Source: CAD feature listing. Evaluate the final solid. Frame: model axes, mm. A direction names the side the tool comes from. Give positions to 0.01 mm unless a question says otherwise; leave off trailing zeros. Order: outer loops, then holes, each group sorted by start corner. A loop starts at its lowest first (then second) coordinate and runs counter-clockwise, first axis right, second up. Notation, with made-up numbers: (61, 4.5) -> (107, 4.5) arc R10 cw to (107, 22.5) -> close; hole circle Ø9 at (42, 1). An arc over 180 degrees is marked (long way). Answer in a Markdown table with one row per item.
```python
from build123d import *

# Parameters (mm, degrees)
F1_DEPTH     = 76.2
F2_R         = 50.0828504331
F2_R_2       = 13.7976444657
F3_DEPTH     = 50.8
F4_T         = -2.54
F5_T3_DEPTH  = 203.2
F5_T5_DEPTH  = 203.2
F5_T8_ANGLE  = 208.0724869359
F5_T10_ANGLE = 151.9275130641


# Not quite as in the source:
# - a fillet or chamfer that OpenCascade refuses, or shapes differently, is made with other operations: its cross-section is extruded or revolved along the edge and cut away or added


with BuildPart() as f1:
    # F0 (on Right) → F1 (new body)
    with BuildSketch(Plane.YZ):
        with BuildLine():
            ThreePointArc((18.4812146278, -73.9248585111), (60.0612543768, -46.8944103565), (76.2, 0))
            ThreePointArc((76.2, 0), (60.0612543768, 46.8944103565), (18.4812146278, 73.9248585111))
            ThreePointArc((18.4812146278, 73.9248585111), (-76.2, 0), (18.4812146278, -73.9248585111))
        make_face()
        with BuildLine():
            ThreePointArc((18.4812146278, 73.9248585111), (60.0612543768, 46.8944103565), (76.2, 0))
            ThreePointArc((76.2, 0), (60.0612543768, -46.8944103565), (18.4812146278, -73.9248585111))
            Line((18.4812146278, -73.9248585111), (215.6141706573, -24.6416195037))
            ThreePointArc((215.6141706573, -24.6416195037), (184.0537657814, 0), (215.6141706573, 24.6416195037))
            Line((215.6141706573, 24.6416195037), (18.4812146278, 73.9248585111))
        make_face()
        with BuildLine():
            ThreePointArc((234.8537657814, 0), (229.474183907, 15.6314701188), (215.6141706573, 24.6416195037))
            ThreePointArc((215.6141706573, 24.6416195037), (184.0537657814, 0), (215.6141706573, -24.6416195037))
            ThreePointArc((215.6141706573, -24.6416195037), (229.474183907, -15.6314701188), (234.8537657814, 0))
        make_face()
    extrude(amount=F1_DEPTH)

    # F2 (on face) → F3 (cut)
    with BuildSketch(Plane.YZ.offset(76.2)):
        Circle(F2_R)
        with Locations((209.4537657814, 0)):
            Circle(F2_R_2)
    extrude(amount=-F3_DEPTH, mode=Mode.SUBTRACT)

    # F4
    f4_openings = [f1.faces().sort_by_distance(p)[0] for p in [
        (0, 57.51924, 0),
    ]]
    offset(amount=F4_T, openings=f4_openings, kind=Kind.INTERSECTION)

    # F5: fillet of radius 6.35 on 7 edges, made by hand

    # F5_s1 → F5_t2 (revolve)
    with BuildSketch(Plane.XY):
        with BuildLine():
            ThreePointArc((31.75, 50.0828504331), (27.2598719395, 48.2229784936), (25.4, 43.7328504331))
            Line((25.4, 43.7328504331), (25.4, 50.0828504331))
            Line((25.4, 50.0828504331), (31.75, 50.0828504331))
        make_face()
    revolve(axis=Axis((25.4, 0, 0), (1, 0, 0)))

    # F5_s4 → F5_t3 (cut)
    with BuildSketch(Plane(origin=(0, 197.1329560295, -49.2832390074), x_dir=(1, 0, 0), z_dir=(0, -0.9701425001, 0.242535625))):
        with BuildLine():
            ThreePointArc((69.85, 76.2), (74.3401280605, 74.3401280605), (76.2, 69.85))
            Line((76.2, 69.85), (76.2, 76.2))
            Line((76.2, 76.2), (69.85, 76.2))
        make_face()
    extrude(amount=F5_T3_DEPTH, mode=Mode.SUBTRACT)

    # F5_s6 → F5_t5 (cut)
    with BuildSketch(Plane(origin=(0, 0, 0), x_dir=(1, 0, 0), z_dir=(0, 0.9701425001, 0.242535625))):
        with BuildLine():
            ThreePointArc((69.85, 76.2), (74.3401280605, 74.3401280605), (76.2, 69.85))
            Line((76.2, 69.85), (76.2, 76.2))
            Line((76.2, 76.2), (69.85, 76.2))
        make_face()
    extrude(amount=F5_T5_DEPTH, mode=Mode.SUBTRACT)

    # F5_s7 → F5_t8 (revolve, cut)
    with BuildSketch(Plane(origin=(0, 0, 0), x_dir=(1, 0, 0), z_dir=(0, 0.9701425001, -0.242535625))):
        with BuildLine():
            ThreePointArc((69.85, -76.2), (74.3401280605, -74.3401280605), (76.2, -69.85))
            Line((76.2, -69.85), (76.2, -76.2))
            Line((76.2, -76.2), (69.85, -76.2))
        make_face()
    revolve(axis=Axis((76.2, 0, 0), (1, 0, 0)), revolution_arc=F5_T8_ANGLE, mode=Mode.SUBTRACT)

    # F5_s9 → F5_t10 (revolve, cut)
    with BuildSketch(Plane(origin=(0, 197.1329560295, 49.2832390074), x_dir=(1, 0, 0), z_dir=(0, -0.9701425001, -0.242535625))):
        with BuildLine():
            ThreePointArc((76.2, -69.85), (74.3401280605, -74.3401280605), (69.85, -76.2))
            Line((69.85, -76.2), (76.2, -76.2))
            Line((76.2, -76.2), (76.2, -69.85))
        make_face()
    revolve(axis=Axis((76.2, 209.4537657814, 0), (1, 0, 0)), revolution_arc=F5_T10_ANGLE, mode=Mode.SUBTRACT)

    # F5_s11 → F5_t12 (revolve, cut)
    with BuildSketch(Plane.XY):
        with BuildLine():
            ThreePointArc((76.2, 56.4328504331), (74.3401280605, 51.9427223726), (69.85, 50.0828504331))
            Line((69.85, 50.0828504331), (76.2, 50.0828504331))
            Line((76.2, 50.0828504331), (76.2, 56.4328504331))
        make_face()
    revolve(axis=Axis((76.2, 0, 0), (1, 0, 0)), mode=Mode.SUBTRACT)

    # F5_s13 → F5_t14 (revolve, cut)
    with BuildSketch(Plane.XY):
        with BuildLine():
            ThreePointArc((76.2, 229.6014102471), (74.3401280605, 225.1112821866), (69.85, 223.2514102471))
            Line((69.85, 223.2514102471), (76.2, 223.2514102471))
            Line((76.2, 223.2514102471), (76.2, 229.6014102471))
        make_face()
    revolve(axis=Axis((76.2, 209.4537657814, 0), (1, 0, 0)), mode=Mode.SUBTRACT)


solid = f1.part
```
(1) Pull-direction query (Y, two-part tool) for faces 1 (the flat face through (0, 79, 57)), 2 (the flat face through (36.314, 115.052, -47.164)), 3 (the flat face through (34.436, 115.668, -49.628)); classes: +Y half, -Y half, draft (parallel to the pull), parting line (faces both ways), or undercut.
A:
| item | result |
|---|---|
| face 1 | draft |
| face 2 | undercut |
| face 3 | +Y half |
(2) Access query for faces 4 (the flat face through (36.314, 117.812, 46.474)), 5 (the cylindrical face through (47.94, 195.67, 0.61)), 6 (the cylindrical face through (74.29, 115.23, -47.87)). Directions: +Z, -Z, +X, -X, +Y, -Y. A direction counts if a zero-diameter tool reaches every point of the face in a straight line with its end or side. Return the directions, or none.
A:
| item | result |
|---|---|
| face 4 | -X |
| face 5 | +X |
| face 6 | -Z, +X, +Y |
(3) Section query C-C (y = 0). Return the cut outline in (x, z).
A:
| item | result |
|---|---|
| outline | (0, -76.2) -> (69.85, -76.2) arc R6.35 ccw to (76.2, -69.85) -> (76.2, -56.43) arc R6.35 ccw to (69.85, -50.08) -> (31.75, -50.08) arc R6.35 cw to (25.4, -43.73) -> (25.4, 43.73) arc R6.35 cw to (31.75, 50.08) -> (69.85, 50.08) arc R6.35 ccw to (76.2, 56.43) -> (76.2, 69.85) arc R6.35 ccw to (69.85, 76.2) -> (0, 76.2) -> (0, 73.66) -> (73.66, 73.66) -> (73.66, 52.62) -> (22.86, 52.62) -> (22.86, -52.62) -> (73.66, -52.62) -> (73.66, -73.66) -> (0, -73.66) -> close |
(4) First-contact query: pin 1 Ø6 at (y, z) = (-1.5, -38) entering from +X; pin 2 Ø8 at (x, z) = (28, -36) entering from -Y; pin 3 Ø12 at (x, y) = (46.5, 170.5) entering from -Z; pin 4 Ø8 at (x, z) = (29, -0.5) entering from -Y. Flat tips, straight axial feed; report the tip coordinate or a pass-through.
A:
| item | result |
|---|---|
| pin 1 | stops at x = 25.4 |
| pin 2 | stops at y = -69.16 |
| pin 3 | stops at z = -37.42 |
| pin 4 | stops at y = -76.2 |
(5) Ray query, probe 1 along Z at (x, y) = (47, 0); probe 2 along Z at (x, y) = (52.5, -6.5); probe 3 along X at (y, z) = (-6, 15). Return the intervals inside material, ascending.
A:
| item | result |
|---|---|
| probe 1 | z = -76.2 to -73.66, -52.62 to -50.08, 50.08 to 52.62, 73.66 to 76.2 |
| probe 2 | z = -75.92 to -73.37, -52.22 to -49.66, 49.66 to 52.22, 73.37 to 75.92 |
| probe 3 | x = 22.86 to 25.4 |
(6) Section query A-A (x = 39). Return the cut outline in (y, z).
A:
| item | result |
|---|---|
| outline | circle Ø105.25 at (0, 0); (18.48, -73.92) -> (215.61, -24.64) arc R25.4 ccw to (215.61, 24.64) -> (18.48, 73.92) arc R76.2 ccw (long way) to start; circle Ø32.68 at (209.45, 0); hole circle Ø100.17 at (0, 0); hole (17.87, -71.46) -> (215, -22.18) arc R22.86 ccw to (215, 22.18) -> (17.87, 71.46) arc R73.66 ccw (long way) to start; hole circle Ø27.6 at (209.45, 0) |
(7) Section query B-B (x = 20). Return the cut outline in (y, z).
A:
| item | result |
|---|---|
| outline | (18.48, -73.92) -> (215.61, -24.64) arc R25.4 ccw to (215.61, 24.64) -> (18.48, 73.92) arc R76.2 ccw (long way) to start; hole (17.87, -71.46) -> (215, -22.18) arc R22.86 ccw to (215, 22.18) -> (17.87, 71.46) arc R73.66 ccw (long way) to start |
